Autodesk Inventor part; units mm, degrees
ref_plane "YZ Plane" through (0, 0, 0) normal (1, 0, 0) x (0, 1, 0)
ref_plane "XZ Plane" through (0, 0, 0) normal (0, 1, 0) x (-1, 0, 0)
ref_plane "XY Plane" through (0, 0, 0) normal (0, 0, 1) x (1, 0, 0)
sketch "Sketch1" plane through (-4.5, -9.15, 9.417) normal (0, -1, 0) x (1, 0, 0)
  point P0 (4.5, -9.417)
sketch "Sketch2" plane through (1.8079, 5.5858, 15) normal (0, 0, 1) x (1, 0, 0)
  line L0 (-1.8079, -5.5858) -> (-1.8079, -0.7733)
  circle A0 centre (-8.2214, -4.4747) radius 6.35
  circle A1 centre (4.6056, -4.4747) radius 6.35
  dimension "d0" = 12.7
  dimension "d1" = 6.4135
  dimension "d2" = 12.7
  dimension "d3" = 6.4135
extrude "Extrusion1" add sketch "Sketch2" along normal mid plane 44.45
sketch "Sketch4" plane through (6.4135, 1.1111, 37.225) normal (0, 0, 1) x (1, 0, 0)
  circle A0 centre (3.175, -10.541) radius 4.445
  circle A1 centre (0, 0) radius 6.35
  point P0 (-6.4135, -1.1111)
  dimension "d7" = 8.89
  dimension "d8" = 10.541
  dimension "d9" = 3.175
sketch "Sketch5" plane through (-6.4135, 1.1111, 37.225) normal (0, 0, 1) x (1, 0, 0)
  circle A0 centre (-3.175, -10.541) radius 4.445
  circle A1 centre (0, 0) radius 6.35
  point P0 (6.4135, -1.1111)
  dimension "d10" = 8.89
  dimension "d11" = 3.175
  dimension "d12" = 10.541
extrude "Extrusion2" add sketch "Sketch4" against normal blind 19.05 contours A0
extrude "Extrusion3" add sketch "Sketch5" against normal blind 19.05 contours A0
sketch "Sketch6" plane through (-9.5885, -9.4299, 37.225) normal (0, 0, 1) x (1, 0, 0)
  circle A0 centre (-8.89, 2.54) radius 4.445
  circle A1 centre (0, 0) radius 4.445
  line L0 (0, 0) -> (0, 2.54)
  point P0 (9.5885, 9.4299)
  dimension "d17" = 8.89
  dimension "d18" = 8.89
  dimension "d52" = 2.54
  dimension "d53" = 0
extrude "Extrusion4" add sketch "Sketch6" against normal blind 19.05 contours A0
sketch "Sketch7" plane through (9.5885, -9.4299, 37.225) normal (0, 0, 1) x (1, 0, 0)
  circle A0 centre (8.89, 2.54) radius 4.445
  circle A1 centre (0, 0) radius 4.445
  line L0 (0, 0) -> (0, 2.54)
  point P0 (-9.5885, 9.4299)
  dimension "d22" = 8.89
  dimension "d54" = 2.54
  dimension "d55" = 0
extrude "Extrusion5" add sketch "Sketch7" against normal blind 19.05 contours A0
sketch "Sketch8" plane through (6.4135, 1.1111, 37.225) normal (0, 0, 1) x (1, 0, 0)
  line L0 (-7.62, -6.7786) -> (7.62, -6.7786)
  line L1 (7.62, -6.7786) -> (7.62, 7.1914)
  line L2 (7.62, 7.1914) -> (-7.62, 7.1914)
  line L3 (-7.62, 7.1914) -> (-7.62, -6.7786)
  line L4 (-7.62, -6.7786) -> (7.62, 7.1914) construction
  line L5 (7.62, -6.7786) -> (-7.62, 7.1914) construction
  point P0 (-6.4135, -1.1111)
  point P1 (0, 0.2064)
  dimension "d27" = 15.24
  dimension "d28" = 13.97
sketch "Sketch9" plane through (-6.4135, 1.1111, 37.225) normal (0, 0, 1) x (1, 0, 0)
  line L0 (-7.62, -6.7768) -> (7.62, -6.7768)
  line L1 (7.62, -6.7768) -> (7.62, 7.1932)
  line L2 (7.62, 7.1932) -> (-7.62, 7.1932)
  line L3 (-7.62, 7.1932) -> (-7.62, -6.7768)
  line L4 (-7.62, -6.7768) -> (7.62, 7.1932) construction
  line L5 (7.62, -6.7768) -> (-7.62, 7.1932) construction
  point P0 (6.4135, -1.1111)
  point P1 (0, 0.2082)
  dimension "d29" = 15.24
  dimension "d30" = 13.97
extrude "Extrusion6" add sketch "Sketch9" along normal blind 1.27
extrude "Extrusion7" add sketch "Sketch8" along normal blind 1.27
sketch "Sketch10" plane through (-6.4135, 1.1111, 38.495) normal (0, 0, 1) x (1, 0, 0)
  line L0 (-7.62, -9.6614) -> (20.447, -9.6614)
  line L1 (20.447, -9.6614) -> (20.447, 7.4393)
  line L2 (20.447, 7.4393) -> (-7.62, 7.4393)
  line L3 (-7.62, 7.4393) -> (-7.62, -9.6614)
  line L4 (-7.62, -9.6614) -> (20.447, 7.4393) construction
  line L5 (20.447, -9.6614) -> (-7.62, 7.4393) construction
  point P0 (6.4135, -1.1111)
extrude "Extrusion8" add sketch "Sketch10" against normal blind 1.27
sketch "Sketch11" plane through (-6.4135, 1.1111, 38.495) normal (0, 0, 1) x (1, 0, 0)
  line L0 (-17.145, -16.0114) -> (1.905, -16.0114)
  line L1 (1.905, -16.0114) -> (1.905, -3.3114)
  line L2 (1.905, -3.3114) -> (-17.145, -3.3114)
  line L3 (-17.145, -3.3114) -> (-17.145, -16.0114)
  line L4 (-7.62, -9.6614) -> (-7.62, 7.4393)
  line L5 (-17.145, -16.0114) -> (1.905, -3.3114) construction
  line L6 (1.905, -16.0114) -> (-17.145, -3.3114) construction
  line L7 (10.922, -16.0114) -> (29.972, -16.0114)
  line L8 (29.972, -16.0114) -> (29.972, -3.3114)
  line L9 (29.972, -3.3114) -> (10.922, -3.3114)
  line L10 (10.922, -3.3114) -> (10.922, -16.0114)
  line L11 (20.447, -9.6614) -> (20.447, 7.4393)
  line L12 (10.922, -16.0114) -> (29.972, -3.3114) construction
  line L13 (29.972, -16.0114) -> (10.922, -3.3114) construction
  line L14 (-12.065, -3.3114) -> (-12.065, 7.4393)
  line L15 (24.892, -3.3114) -> (24.892, 7.4393)
  line L16 (24.892, 7.4393) -> (29.972, -3.3114)
  line L17 (-17.145, -3.3114) -> (-12.065, 7.4393)
  point P0 (6.4135, -1.1111)
  dimension "d37" = 19.05
  dimension "d38" = 12.7
  dimension "d39" = 19.05
  dimension "d40" = 12.7
  dimension "d41" = 5.08
  dimension "d42" = 5.08
extrude "Extrusion9" add sketch "Sketch11" against normal blind 1.27
fillet "Fillet1" radius 0.254 2 edges at (-18.4785, 8.5503, 37.86) (18.4785, 8.5503, 37.86)
fillet "Fillet2" radius 0.254 6 edges at (-14.0335, 8.5503, 37.86) (-18.4785, -2.2003, 37.86) (-14.0335, -2.2003, 37.86) (14.0335, -2.2003, 37.86) (18.4785, -2.2003, 37.86) (14.0335, 8.5503, 37.86)
fillet "Fillet3" radius 3.81 4 edges at (-23.5585, -14.9003, 37.86) (23.5585, -14.9003, 37.86) (-4.5085, -8.5503, 37.86) (4.5085, -8.5503, 37.86)
sketch "Sketch13" plane through (-6.4135, 1.1111, 38.495) normal (0, 0, 1) x (1, 0, 0)
  point P0 (6.4135, -1.1111)
sketch "Sketch14" plane through (-6.4135, 1.1111, 38.495) normal (0, 0, 1) x (1, 0, 0)
  arc A0 (-17.145, -12.2014) -> (-13.335, -16.0114) centre (-13.335, -12.2014) ccw
  line L0 (-17.145, -12.2014) -> (-13.335, -16.0114)
  line L1 (-13.335, -16.0114) -> (-15.2586, -17.935)
  line L2 (-15.2586, -17.935) -> (-19.0686, -14.125)
  line L3 (-19.0686, -14.125) -> (-17.145, -12.2014)
  arc A1 (26.162, -16.0114) -> (29.972, -12.2014) centre (26.162, -12.2014) ccw
  line L4 (26.162, -16.0114) -> (29.972, -12.2014)
  line L5 (29.972, -12.2014) -> (31.5861, -13.8155)
  line L6 (31.5861, -13.8155) -> (27.7761, -17.6255)
  line L7 (27.7761, -17.6255) -> (26.162, -16.0114)
  point P0 (6.4135, -1.1111)
extrude "Extrusion10" cut sketch "Sketch14" against normal blind 1.27 contours L0 A0 | L4 A1
fillet "Fillet4" radius 3.81 4 edges at (-23.5585, -11.0903, 37.86) (-19.7485, -14.9003, 37.86) (23.5585, -11.0903, 37.86) (19.7485, -14.9003, 37.86)
properties part number "Mamba XLX ESC"
The listing builds one solid part. Answer for the finished solid, in the listing's coordinates (mm). A direction names the side the tool comes from. Coordinates: 2 decimals unless noted, no trailing zeros. Loops run counter-clockwise (first coordinate to the right, second up) from the corner with the lowest first, then second, coordinate; pieces in that order, holes last. Notation, with made-up numbers: M 43.25,84 L 53.25,84 A13 ccw 53.25,96 Z; hole C -15.75,46 d3. An arc over 180 degrees is marked long. Answer as a JSON object with one key per item and string values. Group by question number.
Item 1: Section A-A (y = 3.5) is taken. Write down the section's boundary in (x, z) (1 decimal).
Item 2: Which of the six approach directions +Z, -Z, +X, -X, +Y, -Y give full straight-line access (tool end or side, diameter ignored) to faces 1 (the face through (4.508, -14, 38)), 2 (the face through (19.65, -14.6, 37.85)), 3 (the face through (18.478, 3, 38)), 4 (the face through (-21.29, 2.6, 37.87)), 5 (the face through (-14.37, -8.59, 27.83))?
Item 3: Consider L1, parallel to X at y = -10.25, z = 32; L2, parallel to Y at x = -6, z = 10; L3, parallel to X at y = -2.25, z = 3. Determine where each line is inside the solid, lowest interval first.
Item 4: Section C-C (x = -11) is taken. Write down the section's boundary in (y, z) (3 decimals).
Item 5: Each of these flat-tipped pins is pushed along its axis until it touches: P1, Ø0.6, axis at y = 3, z = 38, coming from the -X side; P2, Ø1.4, axis at y = 1, z = 38, coming from the +X side; P3, Ø2.5, axis at x = -10, y = -8.5, coming from the -Z side (3 decimals). Where does it stop, or does it pass through?
Item 6: Section B-B (z = 31) is taken. Give the number of separate pieces and of enclosed holes in the cut face, and give its area (3 significant figures).
Item 7: Section D-D (z = 4.5) is taken. Write down the section's boundary in (x, y).
Item 8: Determine the mould class of faces 6 (the face through (-23.26, -10.99, 37.85)), 7 (the face through (23.558, -6, 38)), 8 (the face through (6.06, -12.13, 27.83)) for opening direction Y: +Y half, -Y half, draft (parallel to the pull), parting line (faces both ways), or undercut.
Solved:
{
 "1": {"outline": "M -20.9,37.2 L -18.5,37.2 L -18.5,38.5 L -20.9,38.5 Z; M -14,37.2 L -12.3,37.2 L -12.3,-7.2 L -0.5,-7.2 L -0.5,37.2 L 0.5,37.2 L 0.5,-7.2 L 12.3,-7.2 L 12.3,37.2 L 14,37.2 L 14,38.5 L -14,38.5 Z; M 18.5,37.2 L 20.9,37.2 L 20.9,38.5 L 18.5,38.5 Z"},
 "2": {"face 1": "+Z, -Z, -Y", "face 2": "+Z, -Z, +X, -Y", "face 3": "+Z, -Z, +Y", "face 4": "+Z, -Z, -X, +Y", "face 5": "-Z"},
 "3": {"L1": "x = -21.39 to -15.57, -13.96 to -5.22, 5.22 to 13.96, 15.57 to 21.39", "L2": "y = -5.23 to 7.45", "L3": "x = -11.8 to -1.03, 1.03 to 11.8"},
 "4": {"outline": "M -14.9,37.225 L -13.645,37.225 L -13.645,18.175 L -5.215,18.175 L -5.215,37.225 L -3.281,37.225 L -3.281,-7.225 L 5.503,-7.225 L 5.503,37.225 L 8.55,37.225 L 8.55,38.495 L -14.9,38.495 Z"},
 "5": {"P1": "stops at x = -21.24", "P2": "stops at x = 22.38", "P3": "stops at z = 18.175"},
 "6": {"separate pieces": "6", "enclosed holes": "0", "area": "502 mm2"},
 "7": {"outline": "C -6.41,1.11 d12.7; C 6.41,1.11 d12.7"},
 "8": {"face 6": "-Y half", "face 7": "draft", "face 8": "undercut"}
}
